from build123d import *

# Parameters (mm, degrees)
CROQUIS1_W              = 50
CROQUIS1_H              = 40
SALIENTE_EXTRUIR1_DEPTH = 7
CROQUIS3_W              = 5.6
CROQUIS3_H              = 5.7
SALIENTE_EXTRUIR3_DEPTH = 50
CROQUIS9_W              = 40
CROQUIS9_H              = 50
SALIENTE_EXTRUIR8_DEPTH = 7
CROQUIS10_W             = 5.7
CROQUIS10_H             = 5.6
SALIENTE_EXTRUIR9_DEPTH = 45
CROQUIS18_W             = 40
CROQUIS18_H             = 6.2
CORTAR_EXTRUIR4_DEPTH   = 5.7
CROQUIS19_W             = 6.2
CROQUIS19_H             = 40
CORTAR_EXTRUIR5_DEPTH   = 5.7
CROQUIS20_R             = 2.5
CORTAR_EXTRUIR6_DEPTH   = 7
CROQUIS21_R             = 2.5
CORTAR_EXTRUIR7_DEPTH   = 7


with BuildPart() as part:
    # Croquis1 → Saliente-Extruir1 (new body)
    with BuildSketch(Plane(origin=(0, 0, 0), x_dir=(1, 0, 0), z_dir=(0, 1, 0))):
        Rectangle(CROQUIS1_W, CROQUIS1_H)
    extrude(amount=SALIENTE_EXTRUIR1_DEPTH)

    # Croquis3 → Saliente-Extruir3 (add)
    with BuildSketch(Plane.ZY.offset(25)):
        with Locations((10, 9.85)):
            Rectangle(CROQUIS3_W, CROQUIS3_H)
        with Locations((-10, 9.85)):
            Rectangle(CROQUIS3_W, CROQUIS3_H)
    extrude(amount=-SALIENTE_EXTRUIR3_DEPTH)

    # Croquis9 → Saliente-Extruir8 (add)
    with BuildSketch(Plane.ZY.offset(25)):
        with Locations((0, -18)):
            Rectangle(CROQUIS9_W, CROQUIS9_H)
    extrude(amount=SALIENTE_EXTRUIR8_DEPTH)

    # Croquis10 → Saliente-Extruir9 (add)
    with BuildSketch(Plane.XZ.offset(43)):
        with Locations((-34.85, 10)):
            Rectangle(CROQUIS10_W, CROQUIS10_H)
        with Locations((-34.85, -10)):
            Rectangle(CROQUIS10_W, CROQUIS10_H)
    extrude(amount=-SALIENTE_EXTRUIR9_DEPTH)

    # Croquis18 → Cortar-Extruir4 (cut)
    with BuildSketch(Plane.ZY.offset(37.7)):
        with Locations((0, -34.1)):
            Rectangle(CROQUIS18_W, CROQUIS18_H)
        with Locations((0, -7.9)):
            Rectangle(CROQUIS18_W, CROQUIS18_H)
    extrude(amount=-CORTAR_EXTRUIR4_DEPTH, mode=Mode.SUBTRACT)

    # Croquis19 → Cortar-Extruir5 (cut)
    with BuildSketch(Plane(origin=(0, 12.7, 0), x_dir=(1, 0, 0), z_dir=(0, 1, 0))):
        with Locations((-13.9, 0)):
            Rectangle(CROQUIS19_W, CROQUIS19_H)
        with Locations((11.1, 0)):
            Rectangle(CROQUIS19_W, CROQUIS19_H)
    extrude(amount=-CORTAR_EXTRUIR5_DEPTH, mode=Mode.SUBTRACT)

    # Croquis20 → Cortar-Extruir6 (cut)
    with BuildSketch(Plane(origin=(0, 7, 0), x_dir=(1, 0, 0), z_dir=(0, 1, 0))):
        with Locations((-13.9, 10)):
            Circle(CROQUIS20_R)
        with Locations((11.1, 10)):
            Circle(CROQUIS20_R)
        with Locations((11.1, -10)):
            Circle(CROQUIS20_R)
        with Locations((-13.9, -10)):
            Circle(CROQUIS20_R)
    extrude(amount=-CORTAR_EXTRUIR6_DEPTH, mode=Mode.SUBTRACT)

    # Croquis21 → Cortar-Extruir7 (cut)
    with BuildSketch(Plane.ZY.offset(32)):
        with Locations((-10, -7.9)):
            Circle(CROQUIS21_R)
        with Locations((10, -7.9)):
            Circle(CROQUIS21_R)
        with Locations((10.339424261, -34.475791146)):
            Circle(CROQUIS21_R)
        with Locations((-10, -34.1)):
            Circle(CROQUIS21_R)
    extrude(amount=-CORTAR_EXTRUIR7_DEPTH, mode=Mode.SUBTRACT)


solid = part.part
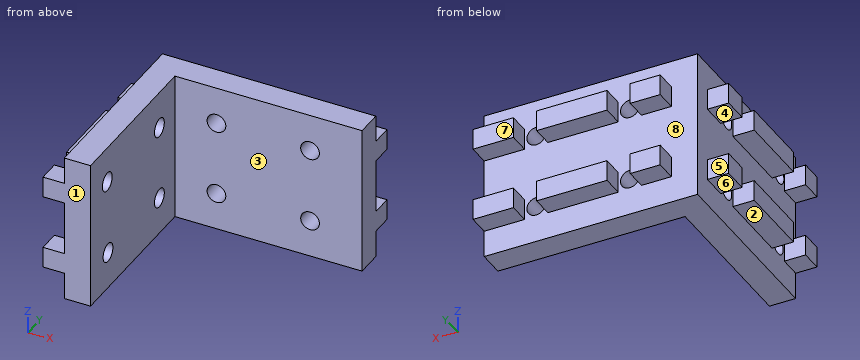
Source: CAD feature listing. Evaluate the final solid. Frame: model axes, mm. Face numbers are marked on the shaded views. A direction names the side the tool comes from. Coordinates: 2 decimals unless noted, no trailing zeros. Order: outer loops, then holes, each group sorted by start corner. A loop starts at its lowest first (then second) coordinate and runs counter-clockwise, first axis right, second up.
Item 1: Material intervals for line 1 (Y direction, x = -27.5, z = -10); line 2 (X direction, y = 5.75, z = 10); line 3 (Z direction, x = -24, y = 10.5), sorted ascending.
Output values:
line 1: y = -43 to -36.6, -31.6 to -10.4, -5.4 to 7
line 2: x = -32 to -16.4, -11.4 to 8.6, 13.6 to 25
line 3: z = -12.8 to -7.2, 7.2 to 12.8
Item 2: Cut plane A-A (x = 11.1). Return loops of the section in (y, z).
Output values:
outline: (0, -20) - (7, -20) - (7, -12.5) - (0, -12.5) - close; (0, -7.5) - (7, -7.5) - (7, 7.5) - (0, 7.5) - close; (0, 12.5) - (7, 12.5) - (7, 20) - (0, 20) - close
Item 3: Set-up query: the marked faces 1, 2, 3, 4 and 5. Return all of +Z, -Z, +X, -X, +Y, -Y with unobstructed straight access to the full face (end or side cutting, diameter ignored); none if empty.
Output values:
face 1: +Z, -Z, +X, -X, -Y
face 2: -Z, -X, +Y, -Y
face 3: +Z, -Z, +X, -Y
face 4: -X, +Y, -Y
face 5: +Z, -Z, -X, +Y
Item 4: Cut plane B-B (y = -7.9). Return loops of the section in (x, z).
Output values:
outline: (-32, -20) - (-25, -20) - (-25, -12.5) - (-32, -12.5) - close; (-32, -7.5) - (-25, -7.5) - (-25, 7.5) - (-32, 7.5) - close; (-32, 12.5) - (-25, 12.5) - (-25, 20) - (-32, 20) - close
Item 5: Cut plane D-D (z = -10). Count the separate pieces of the cut face and the enclosed holes in it, plus the area to 3 significant figures.
Output values:
separate pieces: 5
enclosed holes: 0
area: 960 mm2
Item 6: Cut plane C-C (y = -20.5). Return loops of the section in (x, z).
Output values:
outline: (-37.7, -12.8) - (-32, -12.8) - (-32, -20) - (-25, -20) - (-25, 20) - (-32, 20) - (-32, 12.8) - (-37.7, 12.8) - (-37.7, 7.2) - (-32, 7.2) - (-32, -7.2) - (-37.7, -7.2) - close
Item 7: Pull-direction query (Z, two-part tool) for the marked faces 6, 7 and 8; classes: pulls with the +Z half, pulls with the -Z half, needs draft (parallel to the pull), parting line crosses it, or undercut.
Output values:
face 6: pulls with the -Z half
face 7: needs draft
face 8: undercut
Item 8: First-contact query: P1, Ø3, axis at x = -35.5, y = -41, coming from the +Z side; P2, Ø1, axis at x = 12.5, z = -3.5, coming from the -Y side; P3, Ø4.5, axis at x = -33.5, y = -39, coming from the -Z side; P4, Ø3, axis at x = -35.5, z = -9, coming from the +Y side. Flat tips, straight axial feed; report the tip coordinate or a pass-through.
Output values:
P1: stops at z = 12.8
P2: stops at y = 0
P3: stops at z = -20
P4: stops at y = 2
